Geometry: see drawing. Coordinates: mm, zero at the bounding-box minimum. Round coordinates to 2 decimals unless told otherwise and drop trailing zeros. Loops run counter-clockwise (first coordinate to the right, second up) from the corner with the lowest first, then second, coordinate; pieces in that order, holes last.
(1) Section C-C, the plane x = 9. Return the cut outline in (y, z).
(2) Section B-B, the plane y = 15. Return the cut outline in (x, z).
(3) First-contact query: pin 1 Ø8 at (x, y) = (5, 20.5) entering from +Z; pin 2 Ø1.5 at (x, y) = (20, 15.5) entering from -Z. Flat tips, straight axial feed; report the tip coordinate or a pass-through.
(4) Section D-D, the plane y = 22.5. Return the cut outline in (x, z).
(5) Section A-A, the plane x = 20. Return the cut outline in (y, z).
(6) Material intervals for probe 1 along Y at (x, z) = (20, 2); probe 2 along X at (y, z) = (15, 1.4); probe 3 along Y at (x, z) = (20.5, 1.25) (1 decimal), sorted ascending.
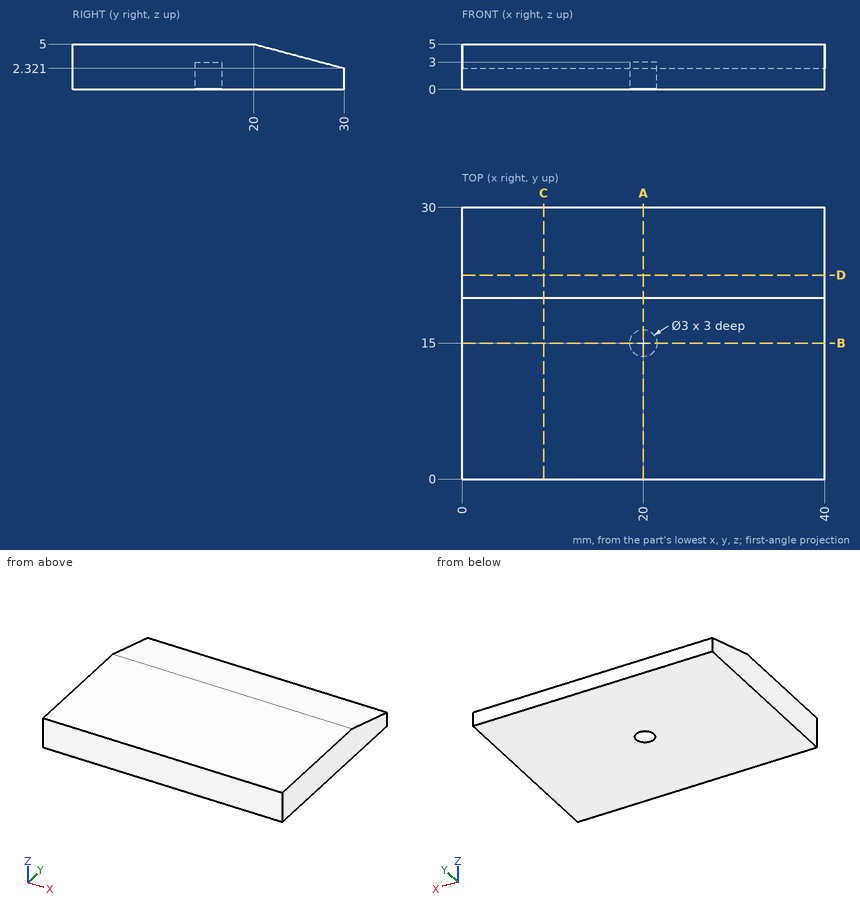
Output values:
1. outline: (0, 0) - (30, 0) - (30, 2.32) - (20, 5) - (0, 5) - close
2. outline: (0, 0) - (18.5, 0) - (18.5, 3) - (21.5, 3) - (21.5, 0) - (40, 0) - (40, 5) - (0, 5) - close
3. pin 1: stops at z = 5
3. pin 2: stops at z = 3
4. outline: (0, 0) - (40, 0) - (40, 4.33) - (0, 4.33) - close
5. outline: (0, 0) - (13.5, 0) - (13.5, 3) - (16.5, 3) - (16.5, 0) - (30, 0) - (30, 2.32) - (20, 5) - (0, 5) - close
6. probe 1: y = 0 to 13.5, 16.5 to 30
6. probe 2: x = 0 to 18.5, 21.5 to 40
6. probe 3: y = 0 to 13.6, 16.4 to 30
